Can you work these out from the model? Positions are in its coordinate system, mm. A direction names the side the tool comes from. Round coordinates to 2 decimals unless told otherwise and drop trailing zeros. Loops run counter-clockwise (first coordinate to the right, second up) from the corner with the lowest first, then second, coordinate; pieces in that order, holes last. Notation, with made-up numbers: (29, 89.5) -> (75, 89.5) arc R34 ccw to (75, 122.5) -> close; hole circle Ø8 at (21.25, 24). An arc over 180 degrees is marked (long way). Write item = value, one per line.
from build123d import *

# Parameters (mm, degrees)
BOSS_EXTRUDE1_DEPTH = 3
BOSS_EXTRUDE2_DEPTH = 20


with BuildPart() as part:
    # Sketch1 → Boss-Extrude1 (new body)
    with BuildSketch(Plane.XY):
        with BuildLine():
            ThreePointArc((3.354101966, 1), (0, 3.5), (-3.354101966, 1))
            Line((-3.354101966, 1), (3.354101966, 1))
        make_face()
        with BuildLine():
            Line((3.354101966, 1), (-3.354101966, 1))
            ThreePointArc((-3.354101966, 1), (-0.505293538, -3.463333429), (3.5, 0))
            ThreePointArc((3.5, 0), (3.463333429, 0.505293538), (3.354101966, 1))
        make_face()
    extrude(amount=BOSS_EXTRUDE1_DEPTH)

    # Sketch2 → Boss-Extrude2 (add)
    with BuildSketch(Plane.XY.offset(3)):
        with BuildLine():
            ThreePointArc((2.015564437, 1), (0, 2.25), (-2.015564437, 1))
            Line((-2.015564437, 1), (2.015564437, 1))
        make_face()
    extrude(amount=BOSS_EXTRUDE2_DEPTH)


solid = part.part
1. I need wall thicknesses on line 1 (Z direction, x = 1.5, y = -1.5); line 2 (Y direction, x = 1.75, z = 20.5); line 3 (Y direction, x = -1.25, z = 19.5). Which ranges of each line are inside material? Lowest first, please. Write a range as [from, to].
Entries:
line_1 = [0, 3]
line_2 = [1, 1.41]
line_3 = [1, 1.87]
2. For faces 1 (the flat face through (0, 1.5, 23)), 2 (the cylindrical face through (0.03, 2.25, 12.86)), 3 (the flat face through (0, 1, 13)), which set-ups out of +Z, -Z, +X, -X, +Y, -Y let a thin tool reach every point of the face, with its end or its side?
Entries:
face_1 = +Z, +X, -X, +Y, -Y
face_2 = +Z, +Y
face_3 = +Z, +X, -X, -Y
3. Suppose I cut it at A-A, the plane x = 0. List the corners of the cut face in (y, z) for me.
Entries:
outline = (-3.5, 0) -> (3.5, 0) -> (3.5, 3) -> (2.25, 3) -> (2.25, 23) -> (1, 23) -> (1, 3) -> (-3.5, 3) -> close
4. I'm going to push a flat-ended pin straight in: pin 1 (2 mm diameter, centred on x = -0.5, z = 14.5, fed in from -Y). Where does the tip first touch, or does it pass through?
Entries:
pin_1 = 1
5. Suppose I cut it at D-D, the plane y = 0.25. List the corners of the cut face in (x, z) for me.
Entries:
outline = (-3.49, 0) -> (3.49, 0) -> (3.49, 3) -> (-3.49, 3) -> close
6. Suppose I cut it at B-B, the plane z = 14.25. List the corners of the cut face in (x, y) for me.
Entries:
outline = (-2.02, 1) -> (2.02, 1) arc R2.25 ccw to start
7. Suppose I cut it at C-C, the plane y = 1.5. List the corners of the cut face in (x, z) for me.
Entries:
outline = (-3.16, 0) -> (3.16, 0) -> (3.16, 3) -> (1.68, 3) -> (1.68, 23) -> (-1.68, 23) -> (-1.68, 3) -> (-3.16, 3) -> close
